Could you check a few things on this drawing? It's one solid part, dimensions in mm from its lowest x, y, z. A direction names the side the tool comes from. Give positions to 0.01 mm unless a question says otherwise; leave off trailing zeros. Loops run counter-clockwise (first coordinate to the right, second up) from the corner with the lowest first, then second, coordinate; pieces in that order, holes last. Notation, with made-up numbers: M 29,80 L 68,80 A23 ccw 68,97 Z; hole C 60.5,-2.5 d10. An arc over 180 degrees is marked long. Write each question's results on one line, items separated by ' | '. Start each with the question number.
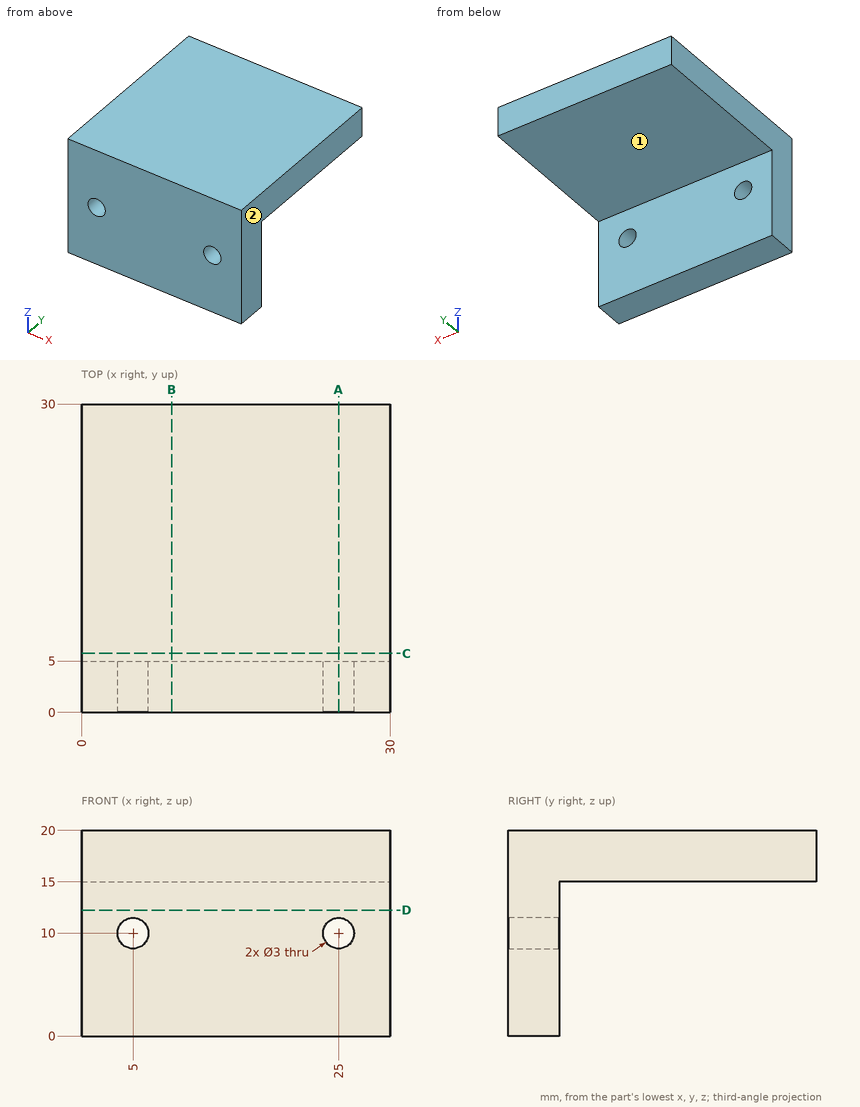
1) If we section it at C-C on y = 5.75: Write out the boundary of the cut face in (x, z), plus the area to 3 significant figures.
2) If we section it at D-D on z = 12.25: Write out the boundary of the cut face in (x, y).
3) Which directions (+Z, -Z, +X, -X, +Y, -Y) give clear straight access to the entire face, cutting with the end or side of a thin tool? Please do the marked faces 1 and 2.
4) Please list where these lines run through material, in increasing order: line 1 (X direction, y = 2.45, z = 10); line 2 (Y direction, x = 16, z = 10); line 3 (Z direction, x = 8.5, y = 19.25). Write a range as from..to.
5) If we section it at B-B on x = 8.75: Write out the boundary of the cut face in (y, z), plus the area to 3 significant figures.
6) I'm going to push flat-ended pins straight in: P1, Ø1.5, axis at x = 7, z = 8, coming from the +Y side; P2, Ø4, axis at x = 15, y = 18, coming from the -Z side. Where does each tip first touch, or does it pass through?
7) If we section it at A-A on x = 25: Write out the boundary of the cut face in (y, z), plus the area to 3 significant figures.
Calculated:
1) outline: M 0,15 L 30,15 L 30,20 L 0,20 Z | area: 150 mm2
2) outline: M 0,0 L 30,0 L 30,5 L 0,5 Z
3) face 1: -Z, +X, -X, +Y | face 2: +Z, -Z, +X, +Y, -Y
4) line 1: x = 0..3.5, 6.5..23.5, 26.5..30 | line 2: y = 0..5 | line 3: z = 15..20
5) outline: M 0,0 L 5,0 L 5,15 L 30,15 L 30,20 L 0,20 Z | area: 225 mm2
6) P1: stops at y = 5 | P2: stops at z = 15
7) outline: M 0,0 L 5,0 L 5,8.5 L 0,8.5 Z; M 0,11.5 L 5,11.5 L 5,15 L 30,15 L 30,20 L 0,20 Z | area: 210 mm2
